Print and shaded views of the part. All mm, measured from the part's lowest x, y and z. Give positions to 0.01 mm unless a question says otherwise; leave off trailing zeros. Loops run counter-clockwise (first coordinate to the right, second up) from the corner with the lowest first, then second, coordinate; pieces in that order, holes last.
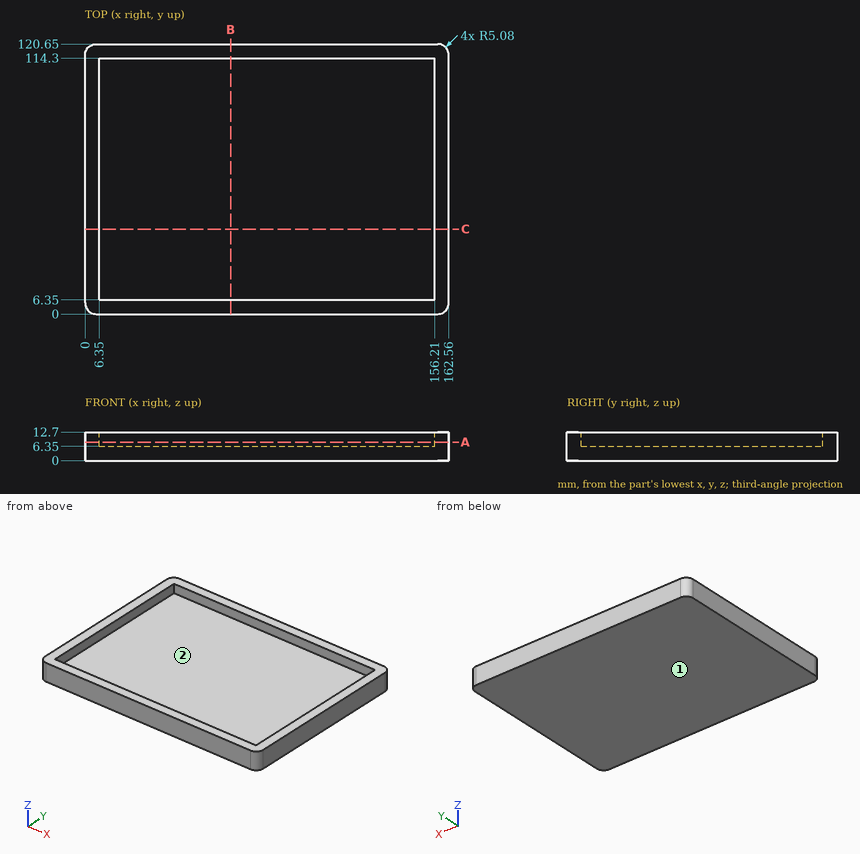
1. Pull direction X, two halves, no side cores. Call the marked faces 1 and 2: released by +X, released by -X, zero draft, split by the parting line, or undercut.
Responses:
face 1: zero draft
face 2: undercut
2. Probe line 1 along X through (y, z) = (30.5, 8.75); line 2 along Y through (x, z) = (87, 10.5); line 3 along Z through (x, y) = (130, 29.5). List the from-to ranges inside material, lowest first.
Responses:
line 1: x = 0 to 6.35, 156.21 to 162.56
line 2: y = 0 to 6.35, 114.3 to 120.65
line 3: z = 0 to 6.35
3. Saw through at A-A, the plane z = 8.25. List the corners of the cut face in (x, y).
Responses:
outline: (0, 5.08) arc R5.08 ccw to (5.08, 0) - (157.48, 0) arc R5.08 ccw to (162.56, 5.08) - (162.56, 115.57) arc R5.08 ccw to (157.48, 120.65) - (5.08, 120.65) arc R5.08 ccw to (0, 115.57) - close; hole (6.35, 6.35) - (156.21, 6.35) - (156.21, 114.3) - (6.35, 114.3) - close
4. Saw through at B-B, the plane x = 65. List the corners of the cut face in (y, z), and give its area (3 significant figures).
Responses:
outline: (0, 0) - (120.65, 0) - (120.65, 12.7) - (114.3, 12.7) - (114.3, 6.35) - (6.35, 6.35) - (6.35, 12.7) - (0, 12.7) - close
area: 847 mm2
5. Drop flat-ended pins along their axis: pin 1 (3 mm diameter, centred on x = 44, y = 82, fed in from +Z); pin 2 (7 mm diameter, centred on y = 75, z = 10, fed in from -X). Give the stop position or say it passes through.
Responses:
pin 1: stops at z = 6.35
pin 2: stops at x = 0
6. Saw through at C-C, the plane y = 38. List the corners of the cut face in (x, z), and give its area (3 significant figures).
Responses:
outline: (0, 0) - (162.56, 0) - (162.56, 12.7) - (156.21, 12.7) - (156.21, 6.35) - (6.35, 6.35) - (6.35, 12.7) - (0, 12.7) - close
area: 1,110 mm2
